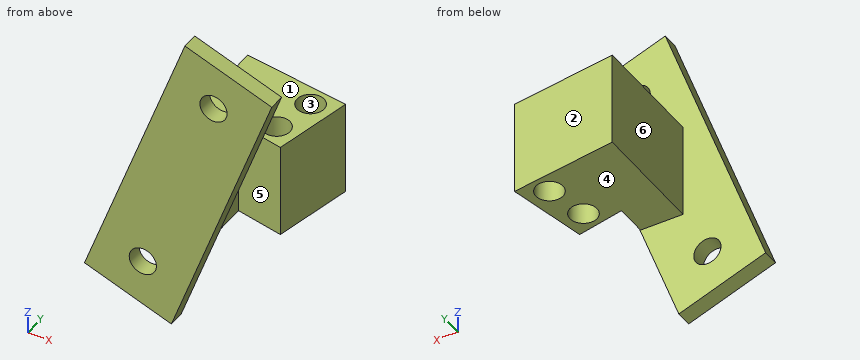
from build123d import *

# Parameters (mm, degrees)
SKETCH1_R            = 3.175
BOSS_EXTRUDE1_DEPTH  = 22.098
SKETCH2_W            = 6.364573253
SKETCH2_H            = 22.098
BOSS_EXTRUDE2_DEPTH  = 8.89
SKETCH12_R           = 3.175
BOSS_EXTRUDE6_DEPTH  = 3.81
BOSS_EXTRUDE12_DEPTH = 22.098
CUT_EXTRUDE1_DEPTH   = 35.052
BOSS_EXTRUDE13_DEPTH = 22.098


with BuildPart() as part:
    # Sketch1 → Boss-Extrude1 (new body)
    with BuildSketch(Plane.XY):
        Polygon((-629.011320926, 228.514758378), (-646.417262265, 232.174381811), (-650.357758597, 213.432549691), (-632.951817258, 209.772926258), align=None)
        with Locations(Location((-635.053635704, 225, 0), (0, 0, 180))):
            Circle(SKETCH1_R, mode=Mode.SUBTRACT)
        with Locations(Location((-637.11116423, 215.213960129, 0), (0, 0, 180))):
            Circle(SKETCH1_R, mode=Mode.SUBTRACT)
    extrude(amount=BOSS_EXTRUDE1_DEPTH)

    # Sketch2 → Boss-Extrude2 (add)
    with BuildSketch(Plane(origin=(15.442364745, 73.44714554, 0), x_dir=(0.9786039871389689, -0.20575285260650125, 0), z_dir=(-0.20575285260650128, -0.978603987138969, 0))):
        with Locations((-677.174764942, 11.049)):
            Rectangle(SKETCH2_W, SKETCH2_H)
    extrude(amount=BOSS_EXTRUDE2_DEPTH)

    # Sketch12 → Boss-Extrude6 (add)
    with BuildSketch(Plane(origin=(0, 204.732760245, 0), x_dir=(1, 0, 0), z_dir=(0, 1, 0))):
        Polygon((-673.35674497, 17.499509084), (-649.901003541, -46.94461085), (-629.613039858, -39.560395955), (-653.068781287, 24.883723978), align=None)
        with Locations(Location((-659.737838472, 11.644339504, 0), (0, 0, 270))):
            Circle(SKETCH12_R, mode=Mode.SUBTRACT)
        with Locations(Location((-643.231946355, -33.705226375, 0), (0, 0, 270))):
            Circle(SKETCH12_R, mode=Mode.SUBTRACT)
    extrude(amount=-BOSS_EXTRUDE6_DEPTH)

    # Sketch19 → Boss-Extrude12 (add)
    with BuildSketch(Plane.XY.offset(22.098)):
        Polygon((-646.417262265, 232.174381811), (-654.037262265, 232.174381811), (-654.037262265, 204.732760245), (-652.186901457, 204.732760245), align=None)
    extrude(amount=-BOSS_EXTRUDE12_DEPTH)

    # Sketch20 → Cut-Extrude1 (cut)
    with BuildSketch(Plane(origin=(0, 0, 0), x_dir=(-1, 0, 0), z_dir=(0, 0, -1))):
        Polygon((629.011320926, 228.514758378), (654.037262265, 232.174381811), (646.417262265, 232.174381811), align=None)
    extrude(amount=-CUT_EXTRUDE1_DEPTH, mode=Mode.SUBTRACT)

    # Sketch21 → Boss-Extrude13 (add)
    with BuildSketch(Plane(origin=(0, 0, 0), x_dir=(-1, 0, 0), z_dir=(0, 0, -1))):
        Polygon((644.129361835, 212.123020588), (644.129361835, 204.732760245), (645.683174376, 204.732760245), align=None)
    extrude(amount=-BOSS_EXTRUDE13_DEPTH)


solid = part.part
Input: part model. Units: mm. Frame: model coordinates. Face numbers are marked on the shaded views. A direction names the side the tool comes from. Coordinates: 2 decimals unless noted, no trailing zeros. Write each loop counter-clockwise with the first axis right and the second up, starting at its lowest first coordinate (ties: lowest second). Pieces come first, ordered by that corner, then holes. Notation, with made-up numbers: M 67.25,-11.75 L 109.25,-11.75 A21 cw 109.25,12.25 Z; hole C 82.5,-5.5 d1. An arc over 180 degrees is marked long. Answer as a JSON object with one key per item and string values. Group by question number.
(1) Section C-C on z = 3.5. Output: boundary loops of the cut face in (x, y) (3 decimals).
(2) Section A-A on y = 211. Output: boundary loops of the cut face in (x, z), plus the area to 3 significant figures.
(3) Set-up query: the marked faces 4, 5 and 6. Return all of +Z, -Z, +X, -X, +Y, -Y with unobstructed straight access to the full face (end or side cutting, diameter ignored); none if empty.
(4) Section D-D on y = 203. Give the number of separate pieces and of enclosed holes in the cut face, plus the area to 3 significant figures.
(5) Section B-B on x = -637.5. Output: boundary loops of the cut face in (y, z), plus the area to 3 significant figures.
(6) Ray query, line 1 along Y through (x, z) = (-637.5, 6); line 2 along Y through (x, z) = (-637, 37); line 3 along X through (y, z) = (225, 13). Return the intervals inside material, ascending. Write a range as [from, to].
(7) Mould query, pull axis X, two halves, no side actions, for the marked faces 1, 2 and 3. Classes: pulls with the +X half, pulls with the -X half, needs draft (parallel to the pull), parting line crosses it, or undercut.
(8) Contact query for flat-ended pins moving along their axis: P1, Ø1, axis at y = 218.5, z = 1, coming from the -X side; P2, Ø13, axis at x = -658, z = 28, coming from the +Y side; P3, Ø6, axis at x = -652.5, y = 213, coming from the -Z side; P4, Ø1, axis at x = -639.5, y = 214.5, coming from the -Z side. Output: stop coordinate, or through.
Result set:
{
 "1": {"outline": "M -665.714,200.923 L -642.738,200.923 L -642.738,204.733 L -644.129,204.733 L -644.129,212.123 L -632.952,209.773 L -629.011,228.515 L -654.037,232.174 L -654.037,204.733 L -665.714,204.733 Z; hole C -637.111,215.214 d6.35; hole C -635.054,225 d6.35"},
 "2": {"outline": "M -654.04,0 L -644.13,0 L -644.13,22.1 L -654.04,22.1 Z; M -638.79,0 L -632.69,0 L -632.69,22.1 L -638.79,22.1 Z", "area": "354 mm2"},
 "3": {"face 4": "-Z, +X, -X, +Y", "face 5": "+Z, -Z", "face 6": "+Z, -Z, -X, +Y"},
 "4": {"separate pieces": "1", "enclosed holes": "2", "area": "1,420 mm2"},
 "5": {"outline": "M 200.92,17.89 L 204.73,17.89 L 204.73,42.43 L 200.92,42.43 Z; M 210.73,0 L 212.06,0 L 212.06,22.1 L 210.73,22.1 Z; M 218.37,0 L 222.98,0 L 222.98,22.1 L 218.37,22.1 Z; M 227.02,0 L 229.76,0 L 229.76,22.1 L 227.02,22.1 Z", "area": "285 mm2"},
 "6": {"line 1": "y = [210.73, 212.06], [218.37, 222.98], [227.02, 229.76]", "line 2": "y = [200.92, 204.73]", "line 3": "x = [-654.04, -638.23], [-631.88, -629.75]"},
 "7": {"face 1": "needs draft", "face 2": "pulls with the +X half", "face 3": "undercut"},
 "8": {"P1": "stops at x = -654.04", "P2": "stops at y = 204.73", "P3": "stops at z = 0", "P4": "passes through"}
}
